CAD build for the part. Positions are in the model's coordinates, mm. A direction names the side the tool comes from. Give positions to 0.01 mm unless a question says otherwise; leave off trailing zeros. Order: outer loops, then holes, each group sorted by start corner. A loop starts at its lowest first (then second) coordinate and runs counter-clockwise, first axis right, second up.
Item 1: Flat gauge pins, fed straight in: P1, Ø3, axis at x = 123, z = 2, coming from the -Y side; P2, Ø6, axis at x = 25, z = -4.5, coming from the -Y side; P3, Ø8, axis at x = 63, y = -8, coming from the +Z side; P4, Ø1.5, axis at x = 30, y = -7.5, coming from the +Z side. Where does each tip first touch, or does it go through?
Item 2: Wall check: L1, parallel to Z at x = 149, y = -4; L2, parallel to Y at x = 176.5, z = 1.25; L3, parallel to Z at x = 34.5, y = -4. Give the ranges that are in metal, low to high.
Item 3: Band-saw the part on A-A on x = 140. Give the cut face in (y, z).
Item 4: Which spindle directions (+Z, -Z, +X, -X, +Y, -Y) get a long thin tool onto all of the face, cutting with end or side? Do faces 4 (the cylindrical face through (132.5, -12.7, 0)), 5 (the cylindrical face through (132.5, 12.7, 0)), 6 (the flat face through (140, 0, 1.588)), 7 (the cylindrical face through (17.24, 6.2, -1.38)), 8 (the flat face through (47.371, 8, -5)). Say none if no direction does.
Item 5: Two-plate mould, pull along X, no slides. Class faces 1 (the cylindrical face through (87.173, -0.176, -2.287)), 2 (the flat face through (141, 0, -1.588)), 3 (the cylindrical face through (59.61, -4.29, -4.68)): released by +X, released by -X, zero draft, split by the parting line, or undercut.
```python
from build123d import *

# Parameters (mm, degrees)
F3_DEPTH = 25.4
F4_DEPTH = 25.4


# Not quite as in the source:
# - ends of sketch curves that miss each other by under 0.0002 mm in the source are joined


with BuildPart() as f1:
    # F0 (on Front) → F1 (revolve)
    with BuildSketch(Plane.XZ):
        with BuildLine():
            Line((0, 4.826), (0, 0))
            Line((0, 0), (184.15, 0))
            Line((184.15, 0), (184.15, 12.7))
            Line((184.15, 12.7), (82.55, 12.7))
            ThreePointArc((82.55, 12.7), (76.9495160289, 8.0259690987), (69.8500007868, 6.350001049))
            Line((69.8500007868, 6.350001049), (49.657, 6.35))
            ThreePointArc((49.657, 6.35), (48.0405538982, 7.0195538982), (47.371, 8.636))
            Line((47.371, 8.636), (47.371, 10.3124))
            Line((47.371, 10.3124), (42.6212, 10.3124))
            ThreePointArc((42.6212, 10.3124), (38.420772371, 7.3825769769), (33.4046742858, 6.35))
            Line((33.4046742858, 6.35), (1.524, 6.35))
            ThreePointArc((1.524, 6.35), (0.4463692655, 5.9036307345), (0, 4.826))
        make_face()
    revolve(axis=Axis((92.075, 0, 0), (1, 0, 0)))

    # F2 (on Front) → F3 (cut)
    with BuildSketch(Plane.XZ):
        with BuildLine():
            Line((189.3032044172, 0), (183.8999837637, 0))
            Line((183.8999837637, 0), (182.3124837637, -1.5875))
            Line((182.3124837637, -1.5875), (98.3069729219, -1.5875))
            ThreePointArc((98.3069729219, -1.5875), (83.7572950904, -2.7862065375), (69.5999860764, -6.35))
            Line((69.5999860764, -6.35), (82.516618073, -56.9406822324))
            Line((82.516618073, -56.9406822324), (124.9158531427, -44.9918061495))
            Line((124.9158531427, -44.9918061495), (189.3032044172, -23.9094942808))
            Line((189.3032044172, -23.9094942808), (189.3032044172, 0))
        make_face()
        with BuildLine():
            Line((182.3124837637, 1.5875), (183.8999837637, 0))
            Line((183.8999837637, 0), (189.3032044172, 0))
            Line((189.3032044172, 0), (189.3032044172, 23.9094942808))
            Line((189.3032044172, 23.9094942808), (183.8999837637, 25.6786675836))
            Line((183.8999837637, 25.6786675836), (124.9158531427, 44.9918061495))
            Line((124.9158531427, 44.9918061495), (82.516618073, 56.9406822324))
            Line((82.516618073, 56.9406822324), (69.5999860764, 6.35))
            ThreePointArc((69.5999860764, 6.35), (83.7572950904, 2.7862065375), (98.3069729219, 1.5875))
            Line((98.3069729219, 1.5875), (182.3124837637, 1.5875))
        make_face()
    extrude(amount=-F3_DEPTH, mode=Mode.SUBTRACT)

    # F2 (on Front) → F4 (cut)
    with BuildSketch(Plane.XZ):
        with BuildLine():
            Line((182.3124837637, 1.5875), (183.8999837637, 0))
            Line((183.8999837637, 0), (189.3032044172, 0))
            Line((189.3032044172, 0), (189.3032044172, 23.9094942808))
            Line((189.3032044172, 23.9094942808), (183.8999837637, 25.6786675836))
            Line((183.8999837637, 25.6786675836), (124.9158531427, 44.9918061495))
            Line((124.9158531427, 44.9918061495), (82.516618073, 56.9406822324))
            Line((82.516618073, 56.9406822324), (69.5999860764, 6.35))
            ThreePointArc((69.5999860764, 6.35), (83.7572950904, 2.7862065375), (98.3069729219, 1.5875))
            Line((98.3069729219, 1.5875), (182.3124837637, 1.5875))
        make_face()
        with BuildLine():
            Line((189.3032044172, 0), (183.8999837637, 0))
            Line((183.8999837637, 0), (182.3124837637, -1.5875))
            Line((182.3124837637, -1.5875), (98.3069729219, -1.5875))
            ThreePointArc((98.3069729219, -1.5875), (83.7572950904, -2.7862065375), (69.5999860764, -6.35))
            Line((69.5999860764, -6.35), (82.516618073, -56.9406822324))
            Line((82.516618073, -56.9406822324), (124.9158531427, -44.9918061495))
            Line((124.9158531427, -44.9918061495), (189.3032044172, -23.9094942808))
            Line((189.3032044172, -23.9094942808), (189.3032044172, 0))
        make_face()
    extrude(amount=F4_DEPTH, mode=Mode.SUBTRACT)


solid = f1.part
```
The answers:
1. P1: stops at y = -12.69
1. P2: stops at y = -6.17
1. P3: stops at z = 4.93
1. P4: passes through
2. L1: z = -1.59 to 1.59
2. L2: y = -12.64 to 12.64
2. L3: z = -4.99 to 4.99
3. outline: (-12.6, -1.59) - (12.6, -1.59) arc R12.7 ccw to (12.6, 1.59) - (-12.6, 1.59) arc R12.7 ccw to start
4. face 4: +X, -X, -Y
4. face 5: +X, -X, +Y
4. face 6: +Z, +X, +Y, -Y
4. face 7: -X
4. face 8: none
5. face 1: released by +X
5. face 2: zero draft
5. face 3: undercut
